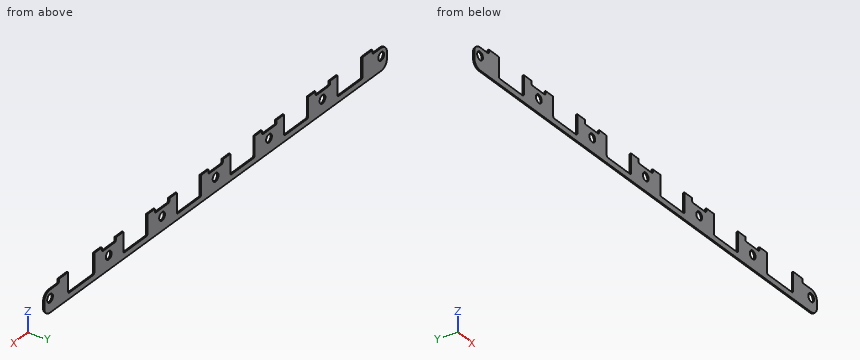
```python
from build123d import *

# Parameters (mm, degrees)
F0_R     = 5
F1_DEPTH = 1.6


with BuildPart() as f1:
    # F0 (on Front) → F1 (new body)
    with BuildSketch(Plane.XZ):
        with BuildLine():
            ThreePointArc((-10, -7), (-7.071068, -14.071068), (0, -17))
            Line((0, -17), (575, -17))
            ThreePointArc((575, -17), (582.071068, -14.071068), (585, -7))
            Line((585, -7), (585, 0))
            ThreePointArc((585, 0), (582.071068, 7.071068), (575, 10))
            Line((575, 10), (561.5, 10))
            ThreePointArc((561.5, 10), (560.085786, 10.585786), (559.5, 12))
            Line((559.5, 12), (559.5, 15))
            Line((559.5, 15), (543.5, 15))
            Line((543.5, 15), (543.5, -8))
            ThreePointArc((543.5, -8), (542.914214, -9.414214), (541.5, -10))
            Line((541.5, -10), (500.25, -10))
            ThreePointArc((500.25, -10), (498.835786, -9.414214), (498.25, -8))
            Line((498.25, -8), (498.25, 15))
            Line((498.25, 15), (485.25, 15))
            Line((485.25, 15), (485.25, 12))
            ThreePointArc((485.25, 12), (484.664214, 10.585786), (483.25, 10))
            Line((483.25, 10), (462.75, 10))
            ThreePointArc((462.75, 10), (461.335786, 10.585786), (460.75, 12))
            Line((460.75, 12), (460.75, 15))
            Line((460.75, 15), (447.75, 15))
            Line((447.75, 15), (447.75, -8))
            ThreePointArc((447.75, -8), (447.164214, -9.414214), (445.75, -10))
            Line((445.75, -10), (408, -10))
            ThreePointArc((408, -10), (406.585786, -9.414214), (406, -8))
            Line((406, -8), (406, 15))
            Line((406, 15), (393, 15))
            Line((393, 15), (393, 12))
            ThreePointArc((393, 12), (392.414214, 10.585786), (391, 10))
            Line((391, 10), (370, 10))
            ThreePointArc((370, 10), (368.585786, 10.585786), (368, 12))
            Line((368, 12), (368, 15))
            Line((368, 15), (355, 15))
            Line((355, 15), (355, -8))
            ThreePointArc((355, -8), (354.414214, -9.414214), (353, -10))
            Line((353, -10), (315.1, -10))
            ThreePointArc((315.1, -10), (313.685786, -9.414214), (313.1, -8))
            Line((313.1, -8), (313.1, 15))
            Line((313.1, 15), (300.1, 15))
            Line((300.1, 15), (300.1, 12))
            ThreePointArc((300.1, 12), (299.514214, 10.585786), (298.1, 10))
            Line((298.1, 10), (277.1, 10))
            ThreePointArc((277.1, 10), (275.685786, 10.585786), (275.1, 12))
            Line((275.1, 12), (275.1, 15))
            Line((275.1, 15), (262.1, 15))
            Line((262.1, 15), (262.1, -8))
            ThreePointArc((262.1, -8), (261.514214, -9.414214), (260.1, -10))
            Line((260.1, -10), (221.85, -10))
            ThreePointArc((221.85, -10), (220.435786, -9.414214), (219.85, -8))
            Line((219.85, -8), (219.85, 15))
            Line((219.85, 15), (206.85, 15))
            Line((206.85, 15), (206.85, 12))
            ThreePointArc((206.85, 12), (206.264214, 10.585786), (204.85, 10))
            Line((204.85, 10), (183.85, 10))
            ThreePointArc((183.85, 10), (182.435786, 10.585786), (181.85, 12))
            Line((181.85, 12), (181.85, 15))
            Line((181.85, 15), (168.85, 15))
            Line((168.85, 15), (168.85, -8))
            ThreePointArc((168.85, -8), (168.264214, -9.414214), (166.85, -10))
            Line((166.85, -10), (129, -10))
            ThreePointArc((129, -10), (127.585786, -9.414214), (127, -8))
            Line((127, -8), (127, 15))
            Line((127, 15), (114, 15))
            Line((114, 15), (114, 12))
            ThreePointArc((114, 12), (113.414214, 10.585786), (112, 10))
            Line((112, 10), (91, 10))
            ThreePointArc((91, 10), (89.585786, 10.585786), (89, 12))
            Line((89, 12), (89, 15))
            Line((89, 15), (76, 15))
            Line((76, 15), (76, -8))
            ThreePointArc((76, -8), (75.414214, -9.414214), (74, -10))
            Line((74, -10), (34.5, -10))
            ThreePointArc((34.5, -10), (33.085786, -9.414214), (32.5, -8))
            Line((32.5, -8), (32.5, 15))
            Line((32.5, 15), (15.5, 15))
            Line((15.5, 15), (15.5, 12))
            ThreePointArc((15.5, 12), (14.914214, 10.585786), (13.5, 10))
            Line((13.5, 10), (0, 10))
            ThreePointArc((0, 10), (-7.071068, 7.071068), (-10, 0))
            Line((-10, 0), (-10, -7))
        make_face()
        Circle(F0_R, mode=Mode.SUBTRACT)
        with Locations((102, 0)):
            Circle(F0_R, mode=Mode.SUBTRACT)
        with Locations((194.85, 0)):
            Circle(F0_R, mode=Mode.SUBTRACT)
        with Locations((287.6, 0)):
            Circle(F0_R, mode=Mode.SUBTRACT)
        with Locations((380.5, 0)):
            Circle(F0_R, mode=Mode.SUBTRACT)
        with Locations((473.25, 0)):
            Circle(F0_R, mode=Mode.SUBTRACT)
        with Locations((575, 0)):
            Circle(F0_R, mode=Mode.SUBTRACT)
    extrude(amount=F1_DEPTH)


solid = f1.part
```
Work out the finished part from the listing and answer in its coordinate system (mm). Round coordinates to 2 decimals unless told otherwise and drop trailing zeros. Loops run counter-clockwise (first coordinate to the right, second up) from the corner with the lowest first, then second, coordinate; pieces in that order, holes last. Notation, with made-up numbers: M 2,37.25 L 37,37.25 A32 cw 37,64.25 Z; hole C -36.75,25.25 d10. An arc over 180 degrees is marked long. Use CSV: the item, a comma, the result in double quotes.
Q1. Consider L1, parallel to Z at x = 473.25, y = -1; L2, parallel to Z at x = 467, y = -0.1; L3, parallel to Z at x = 248, y = -0.95. Determine where each line is inside the solid, lowest interval first.
Determined:
L1,"-17 to -5, 5 to 10"
L2,"-17 to 10"
L3,"-17 to -10"
Q2. Section A-A, the plane x = 473.25 is taken. Determine the outline of the cut face in (y, z), then the cut area to 3 significant figures.
Determined:
outline,"M -1.6,-17 L 0,-17 L 0,-5 L -1.6,-5 Z; M -1.6,5 L 0,5 L 0,10 L -1.6,10 Z"
area,"27.2 mm2"
Q3. Section C-C, the plane x = 139 is taken. Determine the outline of the cut face in (y, z).
Determined:
outline,"M -1.6,-17 L 0,-17 L 0,-10 L -1.6,-10 Z"
Q4. Section B-B, the plane y = -0.7 is taken. State how many separate pieces and enclosed holes the cut face has, then the cut area to 3 significant figures.
Determined:
separate pieces,"1"
enclosed holes,"7"
area,"11,100 mm2"
Q5. Each of these flat-tipped pins is pushed along its axis until it touches: pin 1 (9 mm diameter, centred on x = 473.25, z = 0, fed in from -Y) (3 decimals); pin 2 (0.8 mm diameter, centred on y = -0.5, z = 3.5, fed in from -X); pin 3 (0.5 mm diameter, centred on x = 477.5, y = -1, fed in from +Z); pin 4 (0.8 mm diameter, centred on y = -1, z = 13, fed in from -X). Where does it stop, or does it pass through?
Determined:
pin 1,"through"
pin 2,"x = -9.51"
pin 3,"z = 10"
pin 4,"x = 15.5"
